from build123d import *

# Parameters (mm, degrees)
BOSS_EXTRUDE1_DEPTH         = 25.4
BOSS_EXTRUDE2_DEPTH         = 63.5
CUT_EXTRUDE1_DEPTH          = 51.8
CUT_EXTRUDE1_DEPTH_BACK     = 51.8
F_1_4_0_75_DIAMETER_HOLE1_D = 19.05
SKETCH6_R                   = 31.75
CUT_EXTRUDE2_DEPTH          = 19.05
F_1_4_1_25_DIAMETER_HOLE1_D = 31.75


with BuildPart() as part:
    # Sketch1 → Boss-Extrude1 (new body)
    with BuildSketch(Plane(origin=(0, 0, 0), x_dir=(1, 0, 0), z_dir=(0, 1, 0))):
        with BuildLine():
            Line((-50.8, 0), (-50.8, -31.75))
            ThreePointArc((-50.8, -31.75), (0, -82.55), (50.8, -31.75))
            Line((50.8, -31.75), (50.8, 0))
            Line((50.8, 0), (-50.8, 0))
        make_face()
    extrude(amount=BOSS_EXTRUDE1_DEPTH)

    # Sketch2 → Boss-Extrude2 (add)
    with BuildSketch(Plane(origin=(0, 0, 0), x_dir=(1, 0, 0), z_dir=(0, 1, 0))):
        Polygon((-50.8, 0), (-50.8, 25.4), (-6.805909488, 101.6), (50.8, 101.6), (50.8, 0), align=None)
    extrude(amount=BOSS_EXTRUDE2_DEPTH)

    # Sketch3 → Cut-Extrude1 (cut, two sides)
    with BuildSketch(Plane(origin=(0, 0, 0), x_dir=(0, 0, -1), z_dir=(1, 0, 0))) as cut_extrude1_sk:
        Polygon((76.2, 63.5), (101.6, 63.5), (101.6, 38.1), align=None)
    extrude(amount=CUT_EXTRUDE1_DEPTH, mode=Mode.SUBTRACT)
    extrude(cut_extrude1_sk.sketch, amount=-CUT_EXTRUDE1_DEPTH_BACK, mode=Mode.SUBTRACT)

    # 1/4 (0.75) Diameter Hole1 (through all)
    with Locations(Plane(origin=(0, 63.5, 0), x_dir=(1, 0, 0), z_dir=(0, 1, 0))):
        with Locations((25.4, 50.8)):
            Hole(F_1_4_0_75_DIAMETER_HOLE1_D / 2)

    # Sketch6 → Cut-Extrude2 (cut)
    with BuildSketch(Plane(origin=(0, 63.5, 0), x_dir=(1, 0, 0), z_dir=(0, 1, 0))):
        Circle(SKETCH6_R)
    extrude(amount=-CUT_EXTRUDE2_DEPTH, mode=Mode.SUBTRACT)

    # 1/4 (1.25) Diameter Hole1 (through all)
    with Locations(Plane(origin=(0, 25.4, 0), x_dir=(1, 0, 0), z_dir=(0, 1, 0))):
        with Locations((0, -31.75)):
            Hole(F_1_4_1_25_DIAMETER_HOLE1_D / 2)


solid = part.part
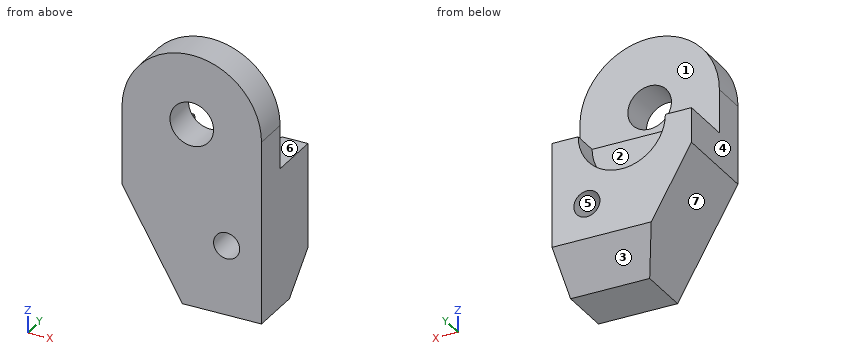
For this review, take the finished solid that the model builds, in its own axes (mm). Face numbers are marked on the shaded views. A direction names the side the tool comes from. Give positions to 0.01 mm unless a question says otherwise; leave off trailing zeros. Loops run counter-clockwise (first coordinate to the right, second up) from the corner with the lowest first, then second, coordinate; pieces in that order, holes last. Notation, with made-up numbers: (28.25, 38) - (64.25, 38) arc R3 ccw to (64.25, 43) - close; hole circle Ø9 at (67.25, -26). An arc over 180 degrees is marked (long way). Write each question's results on one line, items separated by ' | '.
(1) Take a section at A-A (y = 9). Give the boundary of the cut face in (x, z) (3 decimals).
Conclusion:
outline: (-50.8, -25.4) - (-6.806, -101.6) - (50.8, -101.6) - (50.8, 31.75) arc R50.8 ccw to (-50.8, 31.75) - close; hole circle Ø31.75 at (0, 31.75); hole circle Ø19.05 at (25.4, -50.8)
(2) For the marked faces 1, 2 and 3, list the 3-axis set-ups (+Z, -Z, +X, -X, +Y, -Y) from which the entire face can be reached by the end or side of a thin tool; tool diameter is ignored.
Conclusion:
face 1: +Z, +X, -X, +Y | face 2: +Z, +Y | face 3: -Z, +X, -X, +Y
(3) Draft analysis for pull direction Z (two halves, no side actions). For the marked faces 4, 5, 6 and 7, state which applies: +Z half, -Z half, draft (parallel to the pull), parting line (faces both ways), or undercut.
Conclusion:
face 4: draft | face 5: undercut | face 6: +Z half | face 7: -Z half
(4) For line 1 along Z through (x, y) = (0, 13) (3 decimals); line 2 along Z through (x, y) = (25.4, 36) (3 decimals); line 3 along X through (y, z) = (16, 31), list the stretches that pass through material, from the lowest coordinate up.
Conclusion:
line 1: -101.6 to 15.875, 47.625 to 82.55 | line 2: -101.6 to -60.325, -41.275 to 0 | line 3: -50.8 to -15.86, 15.86 to 50.8
(5) Take a section at D-D (z = -50.8). Give the boundary of the cut face in (x, y) (3 decimals), then the cut area to 3 significant figures.
Conclusion:
outline: (-36.135, 0) - (15.875, 0) - (15.875, 63.5) - (-36.135, 63.5) - close; (34.925, 0) - (50.8, 0) - (50.8, 63.5) - (34.925, 63.5) - close | area: 4,310 mm^2
(6) Take a section at C-C (y = 32). Give the boundary of the cut face in (x, z) (3 decimals), then the cut area to 3 significant figures.
Conclusion:
outline: (-50.8, -25.4) - (-6.806, -101.6) - (50.8, -101.6) - (50.8, 0) - (-50.8, 0) - close; hole circle Ø19.05 at (25.4, -50.8) | area: 8,360 mm^2
(7) Take a section at B-B (x = 0). Give the boundary of the cut face in (y, z) (3 decimals).
Conclusion:
outline: (0, -101.6) - (38.1, -101.6) - (63.5, -76.2) - (63.5, -31.75) - (44.45, -31.75) - (44.45, 0) - (25.4, 0) - (25.4, 15.875) - (0, 15.875) - close; (0, 47.625) - (25.4, 47.625) - (25.4, 82.55) - (0, 82.55) - close
(8) For pin 1 Ø8 at (y, z) = (8, -57) entering from -X; pin 2 Ø8 at (x, y) = (-5, 30) entering from +Z; pin 3 Ø4 at (x, y) = (3.5, 46) entering from -Z; pin 4 Ø12 at (x, z) = (9, 29.5) entering from -Y, all flat-tipped, find the tip position at first contact; note any pin that passes through.
Conclusion:
pin 1: x = -34.87 | pin 2: z = 0 | pin 3: z = -95.7 | pin 4: through
